Could you check a few things on this model? Use its own coordinates, in mm. Coordinates: 2 decimals unless noted, no trailing zeros. Loops run counter-clockwise (first coordinate to the right, second up) from the corner with the lowest first, then second, coordinate; pieces in that order, holes last.
from build123d import *

# Parameters (mm, degrees)
SKETCH2_W            = 17.78
SKETCH2_H            = 6.35
CUT_EXTRUDE1_DEPTH   = 12.7
SHELL1_T             = -1.27
SKETCH3_W            = 15.24
SKETCH3_H            = 25.4
BOSS_EXTRUDE1_DEPTH  = 1.5875
M3_CLEARANCE_HOLE1_D = 3.4


with BuildPart() as part:
    # Sketch1 → Revolve1 (revolve)
    with BuildSketch(Plane.XY):
        with BuildLine():
            Line((0, 7.62), (0, -7.62))
            ThreePointArc((0, -7.62), (7.62, 0), (0, 7.62))
        make_face()
    revolve(axis=Axis((0, 7.62, 0), (0, -1, 0)))

    # Sketch2 → Cut-Extrude1 (cut, symmetric)
    with BuildSketch(Plane.XY):
        with Locations((0, 5.715)):
            Rectangle(SKETCH2_W, SKETCH2_H)
    extrude(amount=CUT_EXTRUDE1_DEPTH, both=True, mode=Mode.SUBTRACT)

    # Shell1
    shell1_openings = [part.faces().sort_by_distance(p)[0] for p in [
        (0, 2.54, 0),
    ]]
    offset(amount=SHELL1_T, openings=shell1_openings, kind=Kind.INTERSECTION)

    # Sketch3 → Boss-Extrude1 (add)
    with BuildSketch(Plane(origin=(0, -7.62, 0), x_dir=(1, 0, 0), z_dir=(0, 1, 0))):
        Rectangle(SKETCH3_W, SKETCH3_H)
    extrude(amount=BOSS_EXTRUDE1_DEPTH)

    # M3 Clearance Hole1 (through all)
    with Locations(Plane(origin=(0, -6.0325, 0), x_dir=(1, 0, 0), z_dir=(0, 1, 0))):
        with Locations((-4.445, -9.525), (-4.445, 9.525), (4.445, 9.525), (4.445, -9.525)):
            Hole(M3_CLEARANCE_HOLE1_D / 2)


solid = part.part
1) Imagine slicing it at D-D on z = 2.5. List the corners of the cut face in (x, y) for me.
2) Imagine slicing it at A-A on x = -3.5. List the corners of the cut face in (y, z) for me, plus the area to 3 significant figures.
3) If I drill on L1, parallel to X at y = -3, z = 5; L2, parallel to Z at x = 0, y = 1; L3, parallel to Z at x = -1.75, y = 2, over which ranges is the centre line in solid material (lowest first)?
4) Will these pins go through, and if not, where does the flat tip stop? pin 1 (5 mm diameter, centred on y = 1.5, z = 8.5, fed in from +X); pin 2 (2 mm diameter, centred on x = 3, z = 9, fed in from +Y); pin 3 (6 mm diameter, centred on y = -2, z = -4, fed in from +X); pin 4 (1.5 mm diameter, centred on y = -2.5, z = 9, fed in from -X).
5) We'd pull the mould along Y, two halves only. Please class faces 1 (the flat face through (-5, -6.033, 0)), 2 (the flat face through (0, -6.033, 0)), 3 (the cylindrical face through (3.661, -6.837, 11.033)), 4 (the flat face through (0, -7.62, 0)): released by +Y, released by -Y, zero draft, split by the parting line, or undercut.
6) Imagine slicing it at B-B on z = 9.25. List the corners of the cut face in (x, y) for me.
7) Imagine slicing it at C-C on x = 5. List the corners of the cut face in (y, z) for me.
Solved:
1. outline: (-7.62, -7.62) - (7.62, -7.62) - (7.62, -6.03) - (3.93, -6.03) arc R7.2 ccw to (6.74, 2.54) - (5.26, 2.54) arc R5.84 cw (long way) to (-5.26, 2.54) - (-6.74, 2.54) arc R7.2 ccw to (-3.93, -6.03) - (-7.62, -6.03) - close
2. outline: (-7.62, -12.7) - (-6.03, -12.7) - (-6.03, -10.94) - (-7.62, -10.94) - close; (-7.62, -8.11) - (-6.03, -8.11) - (-6.03, -3.07) arc R6.77 ccw to (2.54, -6.27) - (2.54, -4.65) arc R5.3 cw (long way) to (2.54, 4.65) - (2.54, 6.27) arc R6.77 ccw to (-6.03, 3.07) - (-6.03, 8.11) - (-7.62, 8.11) - close; (-7.62, 10.94) - (-6.03, 10.94) - (-6.03, 12.7) - (-7.62, 12.7) - close
2. area: 63.9 mm2
3. L1: x = -4.91 to -2.51, 2.51 to 4.91
3. L2: z = -7.55 to -6.27, 6.27 to 7.55
3. L3: z = -7.14 to -5.77, 5.77 to 7.14
4. pin 1: stops at x = 4.52
4. pin 2: stops at y = -6.03
4. pin 3: stops at x = 7.48
4. pin 4: passes through
5. face 1: undercut
5. face 2: released by +Y
5. face 3: zero draft
5. face 4: released by -Y
6. outline: (-7.62, -7.62) - (-6.12, -7.62) - (-6.12, -6.03) - (-7.62, -6.03) - close; (-2.77, -7.62) - (2.77, -7.62) - (2.77, -6.03) - (-2.77, -6.03) - close; (6.12, -7.62) - (7.62, -7.62) - (7.62, -6.03) - (6.12, -6.03) - close
7. outline: (-7.62, -12.7) - (-6.03, -12.7) - (-6.03, -11.13) - (-7.62, -11.13) - close; (-7.62, -7.92) - (-6.03, -7.92) - (-6.03, 7.92) - (-7.62, 7.92) - close; (-7.62, 11.13) - (-6.03, 11.13) - (-6.03, 12.7) - (-7.62, 12.7) - close; (2.54, -5.16) - (2.54, -2.98) arc R3.91 cw (long way) to (2.54, 2.98) - (2.54, 5.16) arc R5.75 ccw (long way) to start
